from build123d import *

# Parameters (mm, degrees)
SKETCH1_W           = 14.3
SKETCH1_H           = 5.8
BOSS_EXTRUDE1_DEPTH = 7
SKETCH3_W           = 12
SKETCH3_H           = 4.9
CUT_EXTRUDE1_DEPTH  = 5
SKETCH4_W           = 1.2
SKETCH4_H           = 3.5
CUT_EXTRUDE2_DEPTH  = 4
SKETCH5_W           = 14.3
SKETCH5_H           = 0.8
CUT_EXTRUDE3_DEPTH  = 0.8
SKETCH6_W           = 0.8
SKETCH6_H           = 0.8
CUT_EXTRUDE4_DEPTH  = 10
SKETCH7_W           = 12
SKETCH7_H           = 1
CUT_EXTRUDE5_DEPTH  = 0.3


with BuildPart() as part:
    # Sketch1 → Boss-Extrude1 (new body)
    with BuildSketch(Plane(origin=(0, 0, 0), x_dir=(1, 0, 0), z_dir=(0, 1, 0))):
        Rectangle(SKETCH1_W, SKETCH1_H)
    extrude(amount=BOSS_EXTRUDE1_DEPTH)

    # Sketch3 → Cut-Extrude1 (cut)
    with BuildSketch(Plane.XZ):
        Rectangle(SKETCH3_W, SKETCH3_H)
    extrude(amount=-CUT_EXTRUDE1_DEPTH, mode=Mode.SUBTRACT)

    # Sketch4 → Cut-Extrude2 (cut)
    with BuildSketch(Plane.XY.offset(2.9)):
        with Locations((-3.96, 1.75)):
            Rectangle(SKETCH4_W, SKETCH4_H)
        with Locations((3.94, 1.75)):
            Rectangle(SKETCH4_W, SKETCH4_H)
    extrude(amount=-CUT_EXTRUDE2_DEPTH, mode=Mode.SUBTRACT)

    # Sketch5 → Cut-Extrude3 (cut)
    with BuildSketch(Plane(origin=(0, 7, 0), x_dir=(1, 0, 0), z_dir=(0, 1, 0))):
        with Locations((0, 2.5)):
            Rectangle(SKETCH5_W, SKETCH5_H)
    extrude(amount=-CUT_EXTRUDE3_DEPTH, mode=Mode.SUBTRACT)

    # Sketch6 → Cut-Extrude4 (cut)
    with BuildSketch(Plane(origin=(0, 7, 0), x_dir=(1, 0, 0), z_dir=(0, 1, 0))):
        with Locations((4.3, -0.55)):
            Rectangle(SKETCH6_W, SKETCH6_H)
        with Locations((2.15, -0.55)):
            Rectangle(SKETCH6_W, SKETCH6_H)
        with Locations((0, -0.55)):
            Rectangle(SKETCH6_W, SKETCH6_H)
        with Locations((-2.15, -0.55)):
            Rectangle(SKETCH6_W, SKETCH6_H)
        with Locations((-4.3, -0.55)):
            Rectangle(SKETCH6_W, SKETCH6_H)
    extrude(amount=-CUT_EXTRUDE4_DEPTH, mode=Mode.SUBTRACT)

    # Sketch7 → Cut-Extrude5 (cut)
    with BuildSketch(Plane.XZ.offset(-5)):
        with Locations((0, -1.95)):
            Rectangle(SKETCH7_W, SKETCH7_H)
    extrude(amount=-CUT_EXTRUDE5_DEPTH, mode=Mode.SUBTRACT)


solid = part.part
Source: CAD feature listing. Evaluate the final solid. Frame: model axes, mm. A direction names the side the tool comes from. Round coordinates to 2 decimals unless told otherwise and drop trailing zeros. Loops run counter-clockwise (first coordinate to the right, second up) from the corner with the lowest first, then second, coordinate; pieces in that order, holes last. Notation, with made-up numbers: (69, 65.5) -> (104, 65.5) arc R18 ccw to (104, 90.5) -> close; hole circle Ø4 at (-15.75, 10). An arc over 180 degrees is marked (long way). Answer as a JSON object with one key per item and string values. Group by question number.
Q1. Section query C-C (y = 4.25). Output: boundary loops of the cut face in (x, z).
Q2. Section query A-A (x = -4.25). Output: boundary loops of the cut face in (y, z), plus the area to 3 significant figures.
Q3. Contact query for flat-ended pins moving along their axis: P1, Ø2, axis at x = 2, z = 1, coming from the -Y side; P2, Ø2, axis at x = 3, z = -1.5, coming from the -Y side. Output: stop coordinate, or through.
Q4. Ray query, line 1 (X direction, y = 4.25, z = 2.15); line 2 (Z direction, x = -2.25, y = 6.25); line 3 (X direction, y = 6, z = 0.85). Return the intervals inside material, ascending. Write a range as from..to.
Q5. Section query D-D (z = 1.4). Output: boundary loops of the cut face in (x, y).
Q6. Access query for faces 1 (the flat face through (0, 7, 0)), 2 (the flat face through (0, 5.3, -2)), 3 (the flat face through (-4.3, 6, 0.95)). Directions: +Z, -Z, +X, -X, +Y, -Y. A direction counts if a zero-diameter tool reaches every point of the face in a straight line with its end or side. Return the directions, or none.
Q7. Mould query, pull axis X, two halves, no side actions, for faces 4 (the flat face through (4.3, 6, 0.15)), 5 (the flat face through (0, 3, -2.9)), 6 (the flat face through (-7.15, 3, 0)). Classes: pulls with the +X half, pulls with the -X half, needs draft (parallel to the pull), parting line crosses it, or undercut.
Q8. Section query B-B (y = 6.5). Output: boundary loops of the cut face in (x, z), plus the area to 3 significant figures.
Completed:
{
 "1": {"outline": "(-7.15, -2.9) -> (7.15, -2.9) -> (7.15, 2.9) -> (-7.15, 2.9) -> close; hole (-6, -2.45) -> (6, -2.45) -> (6, 2.45) -> (-6, 2.45) -> close"},
 "2": {"outline": "(0, -2.9) -> (6.2, -2.9) -> (6.2, -2.1) -> (7, -2.1) -> (7, 0.15) -> (5, 0.15) -> (5, -1.45) -> (5.3, -1.45) -> (5.3, -2.45) -> (0, -2.45) -> close; (3.5, 2.45) -> (5, 2.45) -> (5, 0.95) -> (7, 0.95) -> (7, 2.9) -> (3.5, 2.9) -> close", "area": "12.0 mm²"},
 "3": {"P1": "y = 5", "P2": "y = 0"},
 "4": {"line 1": "-7.15..-6, 6..7.15", "line 2": "-2.1..0.15, 0.95..2.9", "line 3": "-7.15..-4.7, -3.9..-2.55, -1.75..-0.4, 0.4..1.75, 2.55..3.9, 4.7..7.15"},
 "5": {"outline": "(-7.15, 0) -> (-6, 0) -> (-6, 5) -> (6, 5) -> (6, 0) -> (7.15, 0) -> (7.15, 7) -> (-7.15, 7) -> close"},
 "6": {"face 1": "+Z, -Z, +X, -X, +Y", "face 2": "-Y", "face 3": "+Y, -Y"},
 "7": {"face 4": "undercut", "face 5": "needs draft", "face 6": "pulls with the -X half"},
 "8": {"outline": "(-7.15, -2.1) -> (7.15, -2.1) -> (7.15, 2.9) -> (-7.15, 2.9) -> close; hole (-4.7, 0.15) -> (-3.9, 0.15) -> (-3.9, 0.95) -> (-4.7, 0.95) -> close; hole (-2.55, 0.15) -> (-1.75, 0.15) -> (-1.75, 0.95) -> (-2.55, 0.95) -> close; hole (-0.4, 0.15) -> (0.4, 0.15) -> (0.4, 0.95) -> (-0.4, 0.95) -> close; hole (1.75, 0.15) -> (2.55, 0.15) -> (2.55, 0.95) -> (1.75, 0.95) -> close; hole (3.9, 0.15) -> (4.7, 0.15) -> (4.7, 0.95) -> (3.9, 0.95) -> close", "area": "68.3 mm²"}
}
